For this review, use the dimensioned drawing (mm, ordinates from the lowest corner) and the shaded views. A direction names the side the tool comes from. Coordinates: 2 decimals unless noted, no trailing zeros. Write each loop counter-clockwise with the first axis right and the second up, starting at its lowest first coordinate (ties: lowest second). Pieces come first, ordered by that corner, then holes.
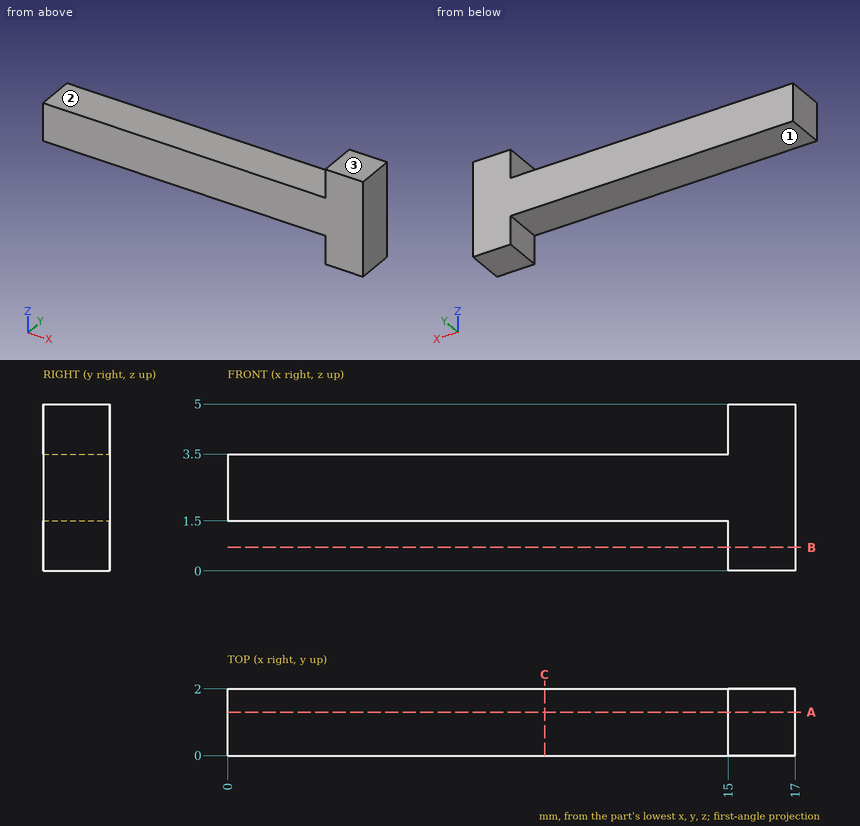
(1) Consider section C-C (x = 9.5). Give the boundary of the cut face in (y, z), plus the area to 3 significant figures.
(2) Consider section B-B (z = 0.7). Give the boundary of the cut face in (x, y), plus the area to 3 significant figures.
(3) Consider section A-A (y = 1.3). Give the boundary of the cut face in (x, z).
(4) Wall thickness on line 1 (X direction, y = 0.8, z = 1.45); line 2 (Z direction, x = 2.5, y = 0.4): over which ranges is each line inside the solid? List them lowest first.
(5) Insertion check: pin 1 Ø0.6 at (x, y) = (5, 1) entering from +Z; pin 2 Ø0.8 at (y, z) = (1.5, 4.5) entering from -X. Each pin has a flat end and moves straight along its axis. Give the tip position at first contact, or say it passes through.
(6) For the marked faces 1, 2 and 3, list the 3-axis set-ups (+Z, -Z, +X, -X, +Y, -Y) from which the entire face can be reached by the end or side of a thin tool; tool diameter is ignored.
Results:
1. outline: (0, 1.5) - (2, 1.5) - (2, 3.5) - (0, 3.5) - close
1. area: 4.00 mm2
2. outline: (15, 0) - (17, 0) - (17, 2) - (15, 2) - close
2. area: 4.00 mm2
3. outline: (0, 1.5) - (15, 1.5) - (15, 0) - (17, 0) - (17, 5) - (15, 5) - (15, 3.5) - (0, 3.5) - close
4. line 1: x = 15 to 17
4. line 2: z = 1.5 to 3.5
5. pin 1: stops at z = 3.5
5. pin 2: stops at x = 15
6. face 1: -Z, -X, +Y, -Y
6. face 2: +Z, -X, +Y, -Y
6. face 3: +Z, +X, -X, +Y, -Y
